Build history of the part. All positions in model axes, mm. Give positions to 0.01 mm unless a question says otherwise; leave off trailing zeros. Order: outer loops, then holes, each group sorted by start corner. A loop starts at its lowest first (then second) coordinate and runs counter-clockwise, first axis right, second up. Notation, with made-up numbers: (18, -39.5) - (69, -39.5) arc R16 ccw to (69, -17.5) - close; hole circle Ø9 at (-17, 83). An arc over 180 degrees is marked (long way). One line per item, written item: value.
```python
from build123d import *

# Parameters (mm, degrees)
SKETCH_1_W               = 82
SKETCH_1_H               = 100
EXTRUDE_1_DEPTH          = 4
SKETCH_2_W               = 82
SKETCH_2_H               = 4
EXTRUDE_2_DEPTH          = 60
CUT_EXTRUDE_1_DEPTH      = 118.460631703
CUT_EXTRUDE_1_DEPTH_BACK = 118.460631703
SKETCH_3_W               = 3
SKETCH_3_H               = 50
CUT_EXTRUDE_2_DEPTH      = 118.460631703
CUT_EXTRUDE_2_DEPTH_BACK = 118.460631703
SKETCH_5_R               = 1.75
CUT_EXTRUDE_3_DEPTH      = 118.460631703
CUT_EXTRUDE_3_DEPTH_BACK = 118.460631703
SKETCH_6_R               = 1.75
CUT_EXTRUDE_4_DEPTH      = 118.460631703
CUT_EXTRUDE_4_DEPTH_BACK = 118.460631703
SKETCH_7_W               = 34
SKETCH_7_H               = 12
FILLET_1_R               = 5
FILLET_2_R               = 2
CUT_EXTRUDE_5_DEPTH      = 118.460631703
CUT_EXTRUDE_5_DEPTH_BACK = 118.460631703
SKETCH_8_R               = 1.75
CUT_EXTRUDE_6_DEPTH      = 118.460631703
CUT_EXTRUDE_6_DEPTH_BACK = 118.460631703
CUT_EXTRUDE_7_DEPTH      = 118.460631703
CUT_EXTRUDE_7_DEPTH_BACK = 118.460631703
SKETCH_10_R              = 1.75


with BuildPart() as part:
    # 草图1 → 凸台-拉伸1 (new body)
    with BuildSketch(Plane(origin=(0, 0, 0), x_dir=(1, 0, 0), z_dir=(0, 1, 0))):
        Rectangle(SKETCH_1_W, SKETCH_1_H)
    extrude(amount=EXTRUDE_1_DEPTH)

    # 草图2 → 凸台-拉伸2 (add)
    with BuildSketch(Plane.XY.offset(50)):
        with Locations((0, 2)):
            Rectangle(SKETCH_2_W, SKETCH_2_H)
    extrude(amount=EXTRUDE_2_DEPTH)

    # 草图3 → 切除-拉伸1 (cut, two sides: drawn at the far end of the back side and taken through both)
    with BuildSketch(Plane(origin=(0, 4, 0), x_dir=(1, 0, 0), z_dir=(0, 1, 0)).offset(-CUT_EXTRUDE_1_DEPTH_BACK)):
        with Locations((-39.5, 25)):
            Rectangle(SKETCH_3_W, SKETCH_3_H)
        with Locations((39.5, 25)):
            Rectangle(SKETCH_3_W, SKETCH_3_H)
        with Locations((-39.5, -85)):
            Rectangle(SKETCH_3_W, SKETCH_3_H)
        with Locations((39.5, -85)):
            Rectangle(SKETCH_3_W, SKETCH_3_H)
    extrude(amount=CUT_EXTRUDE_1_DEPTH + CUT_EXTRUDE_1_DEPTH_BACK, mode=Mode.SUBTRACT)

    # 草图5 → 切除-拉伸2 (cut, two sides: drawn at the far end of the back side and taken through both)
    with BuildSketch(Plane(origin=(0, 4, 0), x_dir=(1, 0, 0), z_dir=(0, 1, 0)).offset(-CUT_EXTRUDE_2_DEPTH_BACK)):
        with Locations(Location((-30, 42, 0), (0, 0, 270))):
            Circle(SKETCH_5_R)
    extrude(amount=CUT_EXTRUDE_2_DEPTH + CUT_EXTRUDE_2_DEPTH_BACK, mode=Mode.SUBTRACT)

    # 草图6 → 切除-拉伸3 (cut, two sides: drawn at the far end of the back side and taken through both)
    with BuildSketch(Plane(origin=(0, 4, 0), x_dir=(1, 0, 0), z_dir=(0, 1, 0)).offset(-CUT_EXTRUDE_3_DEPTH_BACK)):
        with Locations(Location((30, 42, 0), (0, 0, 270))):
            Circle(SKETCH_6_R)
        with Locations(Location((-30, -102, 0), (0, 0, 270))):
            Circle(SKETCH_6_R)
        with Locations(Location((30, -102, 0), (0, 0, 270))):
            Circle(SKETCH_6_R)
    extrude(amount=CUT_EXTRUDE_3_DEPTH + CUT_EXTRUDE_3_DEPTH_BACK, mode=Mode.SUBTRACT)

    # 草图7 → 切除-拉伸4 (cut, two sides: drawn at the far end of the back side and taken through both)
    with BuildSketch(Plane(origin=(0, 4, 0), x_dir=(1, 0, 0), z_dir=(0, 1, 0)).offset(-CUT_EXTRUDE_4_DEPTH_BACK)):
        with Locations((0, -86)):
            Rectangle(SKETCH_7_W, SKETCH_7_H)
        with Locations((0, 26)):
            Rectangle(SKETCH_7_W, SKETCH_7_H)
    extrude(amount=CUT_EXTRUDE_4_DEPTH + CUT_EXTRUDE_4_DEPTH_BACK, mode=Mode.SUBTRACT)

    # 圆角1
    fillet_1_edges = [part.edges().sort_by_distance(p)[0] for p in [
        (38, 2, -50),
        (-38, 2, 110),
        (38, 2, 110),
        (-38, 2, -50),
    ]]
    fillet(fillet_1_edges, radius=FILLET_1_R)

    # 圆角2
    fillet_2_edges = [part.edges().sort_by_distance(p)[0] for p in [
        (41, 2, 0),
        (-41, 2, 60),
        (41, 2, 60),
        (-41, 2, 0),
    ]]
    fillet(fillet_2_edges, radius=FILLET_2_R)

    # 草图8 → 切除-拉伸5 (cut, two sides: drawn at the far end of the back side and taken through both)
    with BuildSketch(Plane(origin=(0, 4, 0), x_dir=(1, 0, 0), z_dir=(0, 1, 0)).offset(-CUT_EXTRUDE_5_DEPTH_BACK)):
        with Locations(Location((0, 42, 0), (0, 0, 270))):
            Circle(SKETCH_8_R)
        with Locations(Location((0, -102, 0), (0, 0, 270))):
            Circle(SKETCH_8_R)
    extrude(amount=CUT_EXTRUDE_5_DEPTH + CUT_EXTRUDE_5_DEPTH_BACK, mode=Mode.SUBTRACT)

    # 草图9 → 切除-拉伸6 (cut, two sides: drawn at the far end of the back side and taken through both)
    with BuildSketch(Plane(origin=(0, 4, 0), x_dir=(1, 0, 0), z_dir=(0, 1, 0)).offset(-CUT_EXTRUDE_6_DEPTH_BACK)):
        with BuildLine():
            Line((20, 33.477548097), (20, 36.477548097))
            Line((20, 36.477548097), (23, 36.477548097))
            Line((23, 36.477548097), (23, 33.477548097))
            ThreePointArc((23, 33.477548097), (21.5, 31.977548097), (20, 33.477548097))
        make_face()
        with BuildLine():
            Line((-23, 36.477548097), (-23, 33.477548097))
            ThreePointArc((-23, 33.477548097), (-21.5, 31.977548097), (-20, 33.477548097))
            Line((-20, 33.477548097), (-20, 36.477548097))
            Line((-20, 36.477548097), (-23, 36.477548097))
        make_face()
        with BuildLine():
            Line((-20, -93.477548097), (-20, -96.477548097))
            Line((-20, -96.477548097), (-23, -96.477548097))
            Line((-23, -96.477548097), (-23, -93.477548097))
            ThreePointArc((-23, -93.477548097), (-21.5, -91.977548097), (-20, -93.477548097))
        make_face()
        with BuildLine():
            Line((23, -96.477548097), (23, -93.477548097))
            ThreePointArc((23, -93.477548097), (21.5, -91.977548097), (20, -93.477548097))
            Line((20, -93.477548097), (20, -96.477548097))
            Line((20, -96.477548097), (23, -96.477548097))
        make_face()
        with BuildLine():
            Line((-20, 18.517447437), (-20, 15.517447437))
            Line((-20, 15.517447437), (-23, 15.517447437))
            Line((-23, 15.517447437), (-23, 18.517447437))
            ThreePointArc((-23, 18.517447437), (-21.5, 20.017447437), (-20, 18.517447437))
        make_face()
        with BuildLine():
            Line((23, 15.517447437), (23, 18.517447437))
            ThreePointArc((23, 18.517447437), (21.5, 20.017447437), (20, 18.517447437))
            Line((20, 18.517447437), (20, 15.517447437))
            Line((20, 15.517447437), (23, 15.517447437))
        make_face()
        with BuildLine():
            Line((20, -78.522451903), (20, -75.522451903))
            Line((20, -75.522451903), (23, -75.522451903))
            Line((23, -75.522451903), (23, -78.522451903))
            ThreePointArc((23, -78.522451903), (21.5, -80.022451903), (20, -78.522451903))
        make_face()
        with BuildLine():
            Line((-23, -75.522451903), (-23, -78.522451903))
            ThreePointArc((-23, -78.522451903), (-21.5, -80.022451903), (-20, -78.522451903))
            Line((-20, -78.522451903), (-20, -75.522451903))
            Line((-20, -75.522451903), (-23, -75.522451903))
        make_face()
    extrude(amount=CUT_EXTRUDE_6_DEPTH + CUT_EXTRUDE_6_DEPTH_BACK, mode=Mode.SUBTRACT)

    # 草图10 → 切除-拉伸7 (cut, two sides: drawn at the far end of the back side and taken through both)
    with BuildSketch(Plane(origin=(0, 4, 0), x_dir=(1, 0, 0), z_dir=(0, 1, 0)).offset(-CUT_EXTRUDE_7_DEPTH_BACK)):
        with Locations(Location((-36.75, -30, 0), (0, 0, 270))):
            Circle(SKETCH_10_R)
        with Locations(Location((36.75, -30, 0), (0, 0, 270))):
            Circle(SKETCH_10_R)
        with Locations(Location((-36.75, -20, 0), (0, 0, 270))):
            Circle(SKETCH_10_R)
        with Locations(Location((36.75, -20, 0), (0, 0, 270))):
            Circle(SKETCH_10_R)
        with Locations(Location((-36.75, -40, 0), (0, 0, 270))):
            Circle(SKETCH_10_R)
        with Locations(Location((36.75, -40, 0), (0, 0, 270))):
            Circle(SKETCH_10_R)
    extrude(amount=CUT_EXTRUDE_7_DEPTH + CUT_EXTRUDE_7_DEPTH_BACK, mode=Mode.SUBTRACT)


solid = part.part
```
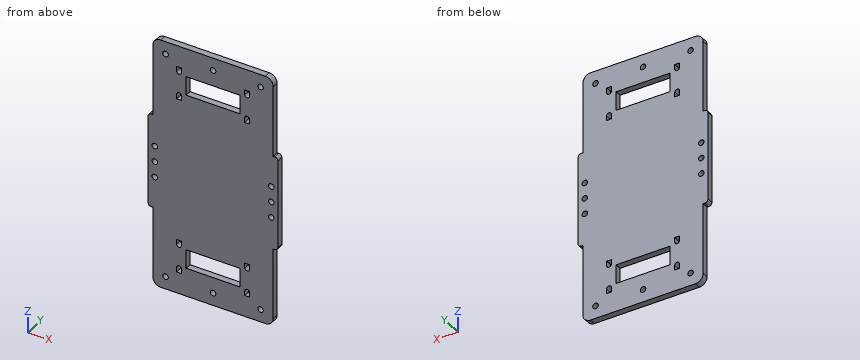
(1) Slice it at B-B, the plane z = 30. Give the cut face in (x, y).
Completed:
outline: (-41, 0) - (-38.5, 0) - (-38.5, 4) - (-41, 4) - close; (-35, 0) - (35, 0) - (35, 4) - (-35, 4) - close; (38.5, 0) - (41, 0) - (41, 4) - (38.5, 4) - close
(2) Slice it at C-C, the plane x = 30. Give the cut face in (y, z).
Completed:
outline: (0, -50) - (4, -50) - (4, -43.75) - (0, -43.75) - close; (0, -40.25) - (4, -40.25) - (4, 100.25) - (0, 100.25) - close; (0, 103.75) - (4, 103.75) - (4, 110) - (0, 110) - close
(3) Drill centre lines: line 1 (Z direction, x = 0, y = 0.9); line 2 (X direction, y = 1.95, z = -42); line 3 (X direction, y = 1.5, z = 30). Where is each one in solid material? Low to high.
Completed:
line 1: -50 to -43.75, -40.25 to -32, -20 to 80, 92 to 100.25, 103.75 to 110
line 2: -38 to -31.75, -28.25 to -1.75, 1.75 to 28.25, 31.75 to 38
line 3: -41 to -38.5, -35 to 35, 38.5 to 41
(4) Slice it at D-D, the plane z = 102. Give the cut face in (x, y), and give its area (3 significant figures).
Completed:
outline: (-38, 0) - (-31.75, 0) - (-31.75, 4) - (-38, 4) - close; (-28.25, 0) - (-1.75, 0) - (-1.75, 4) - (-28.25, 4) - close; (1.75, 0) - (28.25, 0) - (28.25, 4) - (1.75, 4) - close; (31.75, 0) - (38, 0) - (38, 4) - (31.75, 4) - close
area: 262 mm²
(5) Pin check, flat tips, straight feed: P1, Ø0.8, axis at x = 38.5, y = 1.5, coming from the -Z side; P2, Ø0.9, axis at y = 3, z = 95, coming from the -X side; P3, Ø1.5, axis at y = 2.5, z = 77, coming from the +X side; P4, Ø4, axis at x = -36.75, z = 20, coming from the +Y side. Stop position of each tip, or through.
Completed:
P1: z = 0
P2: x = -38
P3: x = 38
P4: y = 4
(6) Slice it at A-A, the plane x = 0. Give the cut face in (y, z).
Completed:
outline: (0, -50) - (4, -50) - (4, -43.75) - (0, -43.75) - close; (0, -40.25) - (4, -40.25) - (4, -32) - (0, -32) - close; (0, -20) - (4, -20) - (4, 80) - (0, 80) - close; (0, 92) - (4, 92) - (4, 100.25) - (0, 100.25) - close; (0, 103.75) - (4, 103.75) - (4, 110) - (0, 110) - close
